Here's how the part is built. I have some questions about the finished solid (model axes, mm). Give positions to 0.01 mm unless a question says otherwise; leave off trailing zeros. Order: outer loops, then holes, each group sorted by start corner. A loop starts at its lowest first (then second) coordinate and runs counter-clockwise, first axis right, second up.
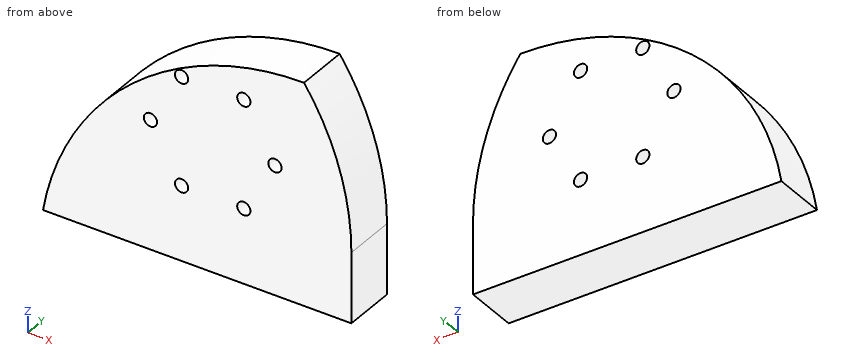
from build123d import *

# Parameters (mm, degrees)
F0_W        = 147.9716226459
F0_H        = 106.0937568545
F1_DEPTH    = 12.7
F2_T1_DEPTH = 651.7371495757
F3_T1_DEPTH = 387.7321882623
F5_D        = 6.35


# Not quite as in the source:
# - a fillet or chamfer that OpenCascade refuses, or shapes differently, is made with other operations: its cross-section is extruded or revolved along the edge and cut away or added


with BuildPart() as f1:
    # F0 (on Front) → F1 (new body, symmetric)
    with BuildSketch(Plane.XZ):
        with Locations((-0.1046992838, -8.5726827383)):
            Rectangle(F0_W, F0_H)
    extrude(amount=F1_DEPTH, both=True)

    # F2: fillet of radius 127 on 1 edges, made by hand

    # F2_s2 → F2_t1 (cut)
    with BuildSketch(Plane.XZ.offset(-325.8685747878)):
        with BuildLine():
            ThreePointArc((51.1769193084, 44.474195689), (-30.9020278112, 14.386766802), (-74.0905106068, -61.6195611656))
            Line((-74.0905106068, -61.6195611656), (-74.0905106068, 44.474195689))
            Line((-74.0905106068, 44.474195689), (51.1769193084, 44.474195689))
        make_face()
    extrude(amount=F2_T1_DEPTH, mode=Mode.SUBTRACT)

    # F3: fillet of radius 127 on 1 edges, made by hand

    # F3_s2 → F3_t1 (cut)
    with BuildSketch(Plane.XZ.offset(-193.8660941311)):
        with BuildLine():
            ThreePointArc((51.1769193084, 44.474195689), (68.0722163397, 9.9776966511), (73.8811120391, -27.9922419635))
            Line((73.8811120391, -27.9922419635), (73.8811120391, 44.474195689))
            Line((73.8811120391, 44.474195689), (51.1769193084, 44.474195689))
        make_face()
    extrude(amount=F3_T1_DEPTH, mode=Mode.SUBTRACT)

    # F5 (through all)
    with Locations(Plane.XZ.offset(12.7)):
        with Locations((-7.6034513134, -25.8695669472), (-22.5392527542, 0), (-7.6034513134, 25.8695669472), (22.2681515682, 25.8695669472), (37.203953009, 0), (22.2681515682, -25.8695669472)):
            Hole(F5_D / 2)


solid = f1.part
Q1. If we section it at C-C on y = -6: List the corners of the cut face in (x, z) for me (3 decimals).
Filled sheet:
outline: (-74.091, -61.62) - (73.881, -61.62) - (73.881, -27.992) arc R127 ccw to (51.177, 44.474) arc R127 ccw to start; hole circle Ø6.35 at (-22.539, 0); hole circle Ø6.35 at (-7.603, -25.87); hole circle Ø6.35 at (-7.603, 25.87); hole circle Ø6.35 at (22.268, -25.87); hole circle Ø6.35 at (22.268, 25.87); hole circle Ø6.35 at (37.204, 0)
Q2. If we section it at B-B on z = 0: List the corners of the cut face in (x, y) for me, plus the area to 3 significant figures.
Filled sheet:
outline: (-45.36, -12.7) - (-25.71, -12.7) - (-25.71, 12.7) - (-45.36, 12.7) - close; (-19.36, -12.7) - (34.03, -12.7) - (34.03, 12.7) - (-19.36, 12.7) - close; (40.38, -12.7) - (70.76, -12.7) - (70.76, 12.7) - (40.38, 12.7) - close
area: 2,630 mm2
Q3. I'm going to push flat-ended pins straight in: P1, Ø2, axis at y = -8, z = -16, coming from the +X side; P2, Ø4, axis at x = 22.27, z = -25.87, coming from the -Y side; P3, Ø3, axis at y = -7.5, z = -3.5, coming from the +X side; P4, Ø1, axis at y = 8, z = -9, coming from the +X side. Where does each tip first touch, or does it pass through?
Filled sheet:
P1: stops at x = 73.4
P2: passes through
P3: stops at x = 71.78
P4: stops at x = 72.53
Q4. I need wall thicknesses on L1, parallel to X at y = 10.75, z = 25; L2, parallel to Z at x = -10.5, y = -5.25; L3, parallel to Z at x = 37, y = -3.75. Which ranges of each line are inside material? Lowest first, please.
Filled sheet:
L1: x = -16.4 to -10.66, -4.55 to 19.21, 25.32 to 62.3
L2: z = -61.62 to -27.17, -24.57 to 24.57, 27.17 to 28.49
L3: z = -61.62 to -3.17, 3.17 to 43.68
Q5. If we section it at D-D on x = 38.5: List the corners of the cut face in (y, z) for me.
Filled sheet:
outline: (-12.7, -61.62) - (12.7, -61.62) - (12.7, -2.9) - (-12.7, -2.9) - close; (-12.7, 2.9) - (12.7, 2.9) - (12.7, 43.84) - (-12.7, 43.84) - close
Q6. If we section it at A-A on x = 21.5: List the corners of the cut face in (y, z) for me.
Filled sheet:
outline: (-12.7, -61.62) - (12.7, -61.62) - (12.7, -28.95) - (-12.7, -28.95) - close; (-12.7, -22.79) - (12.7, -22.79) - (12.7, 22.79) - (-12.7, 22.79) - close; (-12.7, 28.95) - (12.7, 28.95) - (12.7, 40.96) - (-12.7, 40.96) - close
